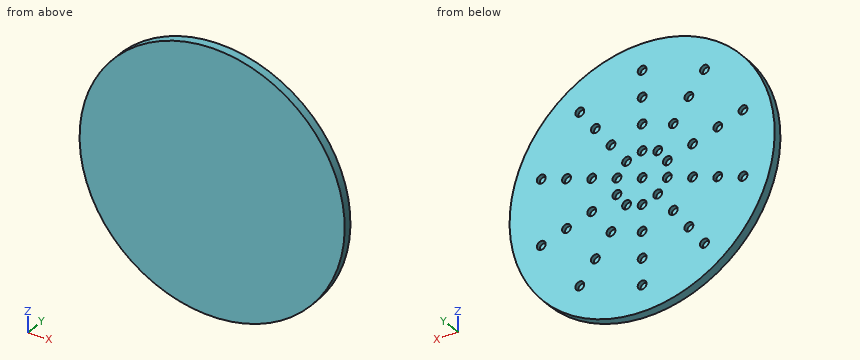
```python
from build123d import *

# Parameters (mm, degrees)
SKETCH1_R           = 381
BOSS_EXTRUDE1_DEPTH = 12.7
SKETCH2_R           = 12.7
CUT_EXTRUDE1_DEPTH  = 12.7


with BuildPart() as part:
    # Sketch1 → Boss-Extrude1 (new, symmetric)
    with BuildSketch(Plane(origin=(0, 0, 0), x_dir=(1, 0, 0), z_dir=(0, 1, 0))):
        with Locations(Location((0, 0, 0), (0, 0, 270))):
            Circle(SKETCH1_R)
    extrude(amount=BOSS_EXTRUDE1_DEPTH, both=True)

    # Sketch2 → Cut-Extrude1 (cut)
    with BuildSketch(Plane(origin=(0, 12.7, 0), x_dir=(1, 0, 0), z_dir=(0, 1, 0))):
        with Locations(Location((0, 304.8, 0), (0, 0, 270))):
            Circle(SKETCH2_R)
        with Locations(Location((-179.156944899, 246.588379885, 0), (0, 0, 270))):
            Circle(SKETCH2_R)
        with Locations(Location((-289.882026167, 94.188379885, 0), (0, 0, 270))):
            Circle(SKETCH2_R)
        with Locations(Location((-289.882026167, -94.188379886, 0), (0, 0, 270))):
            Circle(SKETCH2_R)
        with Locations(Location((-179.156944899, -246.588379886, 0), (0, 0, 270))):
            Circle(SKETCH2_R)
        with Locations(Location((0, -304.8, 0), (0, 0, 270))):
            Circle(SKETCH2_R)
        with Locations(Location((179.156944899, -246.588379885, 0), (0, 0, 270))):
            Circle(SKETCH2_R)
        with Locations(Location((289.882026167, -94.188379885, 0), (0, 0, 270))):
            Circle(SKETCH2_R)
        with Locations(Location((289.882026167, 94.188379886, 0), (0, 0, 270))):
            Circle(SKETCH2_R)
        with Locations(Location((179.156944899, 246.588379886, 0), (0, 0, 270))):
            Circle(SKETCH2_R)
        with Locations(Location((0, 228.6, 0), (0, 0, 270))):
            Circle(SKETCH2_R)
        with Locations(Location((0, 152.4, 0), (0, 0, 270))):
            Circle(SKETCH2_R)
        with Locations(Location((0, 76.2, 0), (0, 0, 270))):
            Circle(SKETCH2_R)
        with Locations(Location((0, 0, 0), (0, 0, 270))):
            Circle(SKETCH2_R)
        with Locations(Location((-134.367708674, 184.941284914, 0), (0, 0, 270))):
            Circle(SKETCH2_R)
        with Locations(Location((-89.578472449, 123.294189943, 0), (0, 0, 270))):
            Circle(SKETCH2_R)
        with Locations(Location((-44.789236225, 61.647094971, 0), (0, 0, 270))):
            Circle(SKETCH2_R)
        with Locations(Location((-217.411519625, 70.641284914, 0), (0, 0, 270))):
            Circle(SKETCH2_R)
        with Locations(Location((-144.941013083, 47.094189943, 0), (0, 0, 270))):
            Circle(SKETCH2_R)
        with Locations(Location((-72.470506542, 23.547094971, 0), (0, 0, 270))):
            Circle(SKETCH2_R)
        with Locations(Location((-217.411519625, -70.641284914, 0), (0, 0, 270))):
            Circle(SKETCH2_R)
        with Locations(Location((-144.941013083, -47.094189943, 0), (0, 0, 270))):
            Circle(SKETCH2_R)
        with Locations(Location((-72.470506542, -23.547094971, 0), (0, 0, 270))):
            Circle(SKETCH2_R)
        with Locations(Location((-134.367708674, -184.941284914, 0), (0, 0, 270))):
            Circle(SKETCH2_R)
        with Locations(Location((-89.578472449, -123.294189943, 0), (0, 0, 270))):
            Circle(SKETCH2_R)
        with Locations(Location((-44.789236225, -61.647094971, 0), (0, 0, 270))):
            Circle(SKETCH2_R)
        with Locations(Location((0, -228.6, 0), (0, 0, 270))):
            Circle(SKETCH2_R)
        with Locations(Location((0, -152.4, 0), (0, 0, 270))):
            Circle(SKETCH2_R)
        with Locations(Location((0, -76.2, 0), (0, 0, 270))):
            Circle(SKETCH2_R)
        with Locations(Location((134.367708674, -184.941284914, 0), (0, 0, 270))):
            Circle(SKETCH2_R)
        with Locations(Location((89.578472449, -123.294189943, 0), (0, 0, 270))):
            Circle(SKETCH2_R)
        with Locations(Location((44.789236225, -61.647094971, 0), (0, 0, 270))):
            Circle(SKETCH2_R)
        with Locations(Location((217.411519625, -70.641284914, 0), (0, 0, 270))):
            Circle(SKETCH2_R)
        with Locations(Location((144.941013083, -47.094189943, 0), (0, 0, 270))):
            Circle(SKETCH2_R)
        with Locations(Location((72.470506542, -23.547094971, 0), (0, 0, 270))):
            Circle(SKETCH2_R)
        with Locations(Location((217.411519625, 70.641284914, 0), (0, 0, 270))):
            Circle(SKETCH2_R)
        with Locations(Location((144.941013083, 47.094189943, 0), (0, 0, 270))):
            Circle(SKETCH2_R)
        with Locations(Location((72.470506542, 23.547094971, 0), (0, 0, 270))):
            Circle(SKETCH2_R)
        with Locations(Location((134.367708674, 184.941284914, 0), (0, 0, 270))):
            Circle(SKETCH2_R)
        with Locations(Location((89.578472449, 123.294189943, 0), (0, 0, 270))):
            Circle(SKETCH2_R)
        with Locations(Location((44.789236225, 61.647094971, 0), (0, 0, 270))):
            Circle(SKETCH2_R)
    extrude(amount=-CUT_EXTRUDE1_DEPTH, mode=Mode.SUBTRACT)


solid = part.part
```
Input: part model. Units: mm. Frame: model coordinates. Give positions to 0.01 mm unless a question says otherwise; leave off trailing zeros. Loops run counter-clockwise (first coordinate to the right, second up) from the corner with the lowest first, then second, coordinate; pieces in that order, holes last.
1) Section query B-B on z = 152.4. Return the cut outline in (x, y).
A:
outline: (-349.19, -12.7) - (349.19, -12.7) - (349.19, 12.7) - (12.7, 12.7) - (12.7, 0) - (-12.7, 0) - (-12.7, 12.7) - (-349.19, 12.7) - close
2) Contact query for flat-ended pins moving along their axis: pin 1 (23 mm diameter, centred on x = -289.88, z = 94.19, fed in from +Y); pin 2 (20.5 mm diameter, centred on x = 84, z = -122.5, fed in from +Y); pin 3 (8 mm diameter, centred on x = -238.5, y = -6.5, fed in from -Z); pin 4 (12 mm diameter, centred on y = -0.5, z = -170, fed in from -X). Output: stop coordinate, or through.
A:
pin 1: stops at y = 0
pin 2: stops at y = 12.7
pin 3: stops at z = -300.28
pin 4: stops at x = -343.9
3) Section query C-C on z = 335.5. Return the cut outline in (x, y), and give its area (3 significant figures).
A:
outline: (-180.56, -12.7) - (180.56, -12.7) - (180.56, 12.7) - (-180.56, 12.7) - close
area: 9,170 mm2
4) Section query A-A on z = -304.8. Return the cut outline in (x, y).
A:
outline: (-228.6, -12.7) - (228.6, -12.7) - (228.6, 12.7) - (12.7, 12.7) - (12.7, 0) - (-12.7, 0) - (-12.7, 12.7) - (-228.6, 12.7) - close
5) Line query: L1, parallel to X at y = 2.5, z = -66.5; L2, parallel to X at y = 11.25, z = -254; L3, parallel to X at y = 7, z = -179.5. Output: solid intervals per line, ascending.
A:
L1: x = -375.15 to -229.42, -205.41 to -56.53, -33.05 to -8.2, 8.2 to 33.05, 56.53 to 205.41, 229.42 to 375.15
L2: x = -283.98 to -189.47, -168.84 to 168.84, 189.47 to 283.98
L3: x = -336.07 to -145.84, -122.89 to 122.89, 145.84 to 336.07
